Check sheet for the modelled part. Datum: model origin and axes. Units: mm. A direction names the side the tool comes from. Coordinates: 2 decimals unless noted, no trailing zeros.
from build123d import *

# Parameters (mm, degrees)
SKETCH_1_W                = 35
SKETCH_1_H                = 5
HOLE_WIZARD_1_D           = 3.4
HOLE_WIZARD_1_DEPTH       = 5
HOLE_WIZARD_2_D           = 52
HOLE_WIZARD_2_DEPTH       = 5
HOLE_WIZARD_2_CBORE_D     = 58.1
HOLE_WIZARD_2_CBORE_DEPTH = 4
HOLE_WIZARD_3_D           = 3.4
HOLE_WIZARD_3_DEPTH       = 5
HOLE_WIZARD_3_CBORE_D     = 6.1
HOLE_WIZARD_3_CBORE_DEPTH = 3
CHAMFER_1_SIZE            = 1
SKETCH_8_R                = 2.2
CUT_EXTRUDE_1_DEPTH       = 3.5


with BuildPart() as part:
    # 草图1 → 旋转1 (revolve)
    with BuildSketch(Plane(origin=(0, 0, 0), x_dir=(1, 0, 0), z_dir=(0, 1, 0))):
        with Locations((17.5, 2.5)):
            Rectangle(SKETCH_1_W, SKETCH_1_H)
    revolve(axis=Axis((0, 0, -5), (0, 0, 1)))

    # 孔1
    with Locations(Plane(origin=(0, 0, -5), x_dir=(-1, 0, 0), z_dir=(0, 0, -1))):
        with Locations((16, -27.712812921), (-16, -27.712812921), (-27.712812921, -16), (-27.712812921, 16), (-16, 27.712812921), (16, 27.712812921), (27.712812921, 16), (27.712812921, -16)):
            Hole(HOLE_WIZARD_1_D / 2, depth=HOLE_WIZARD_1_DEPTH)

    # 孔2
    with Locations(Plane(origin=(0, 0, -5), x_dir=(-1, 0, 0), z_dir=(0, 0, -1))):
        with Locations((0, 0)):
            CounterBoreHole(HOLE_WIZARD_2_D / 2, HOLE_WIZARD_2_CBORE_D / 2, HOLE_WIZARD_2_CBORE_DEPTH, depth=HOLE_WIZARD_2_DEPTH)

    # 孔3
    with Locations(Plane.XY):
        with Locations((0, -32), (0, 32), (-32, 0), (32, 0)):
            CounterBoreHole(HOLE_WIZARD_3_D / 2, HOLE_WIZARD_3_CBORE_D / 2, HOLE_WIZARD_3_CBORE_DEPTH, depth=HOLE_WIZARD_3_DEPTH)

    # 倒角1
    chamfer_1_edges = [part.edges().sort_by_distance(p)[0] for p in [
        (-24.748737342, 24.748737342, 0),
        (24.748737342, -24.748737342, 0),
        (24.748737342, 24.748737342, 0),
        (-24.748737342, -24.748737342, 0),
    ]]
    chamfer(chamfer_1_edges, length=CHAMFER_1_SIZE)

    # 草图8 → 切除-拉伸1 (cut)
    with BuildSketch(Plane(origin=(0, 0, -5), x_dir=(-1, 0, 0), z_dir=(0, 0, -1))):
        with Locations((-27.712812921, 16)):
            Circle(SKETCH_8_R)
        with Locations((-16, 27.712812921)):
            Circle(SKETCH_8_R)
        with Locations((16, 27.712812921)):
            Circle(SKETCH_8_R)
        with Locations((27.712812921, 16)):
            Circle(SKETCH_8_R)
        with Locations((27.712812921, -16)):
            Circle(SKETCH_8_R)
        with Locations((16, -27.712812921)):
            Circle(SKETCH_8_R)
        with Locations((-16, -27.712812921)):
            Circle(SKETCH_8_R)
        with Locations((-27.712812921, -16)):
            Circle(SKETCH_8_R)
    extrude(amount=-CUT_EXTRUDE_1_DEPTH, mode=Mode.SUBTRACT)


solid = part.part
(1) Thickness scan on probe 1 along X at (y, z) = (-18, -4.1); probe 2 along X at (y, z) = (15.5, -4.65); probe 3 along Y at (x, z) = (29.5, -4.4). Record the ranges inside material, lowest first.
Filled in:
probe 1: x = -30.02 to -28.63, -26.8 to -22.8, 22.8 to 26.8, 28.63 to 30.02
probe 2: x = -31.38 to -29.86, -25.57 to -24.57, 24.57 to 25.57, 29.86 to 31.38
probe 3: y = -18.83 to -17.28, -14.72 to 14.72, 17.28 to 18.83
(2) Cross-section at A-A (x = -16). Count the separate pieces of the cut face and the enclosed holes in it, and give its area (3 significant figures).
Filled in:
separate pieces: 4
enclosed holes: 0
area: 34.2 mm2
(3) Go/stop test with flat-tipped pins: P1, Ø2, axis at x = 26.5, z = -3, coming from the +Y side; P2, Ø3, axis at x = -27.5, y = -0.5, coming from the -Z side; P3, Ø2.5, axis at x = -27.71, y = 16, coming from the -Z side; P4, Ø3.5, axis at x = -16, y = -27.71, coming from the -Z side. Record where each tip stops, or that it passes through.
Filled in:
P1: stops at y = 23.97
P2: stops at z = -1
P3: passes through
P4: stops at z = -1.5
(4) Release check for a two-part mould opening along X. For faces 4 (the cylindrical face through (-28, -21, -3)), 5 (the cylindrical face through (0.37, -33.66, -4.01)), 6 (the conical face through (-24.42, -23.9, -0.17)) record: +X half, -X half, draft (parallel to the pull), parting line (faces both ways), or undercut.
Filled in:
face 4: parting line
face 5: undercut
face 6: -X half
(5) Tool access check on faces 1 (the flat face through (15, 26, -1.5)), 2 (the cylindrical face through (29.283, -16.651, -0.739)), 3 (the flat face through (1.31, -30.65, -3)). Record the directions out of +Z, -Z, +X, -X, +Y, -Y that give a thin tool (end or side, any length) a straight path to the whole face; none if there is none.
Filled in:
face 1: -Z
face 2: +Z, -Z
face 3: +Z
